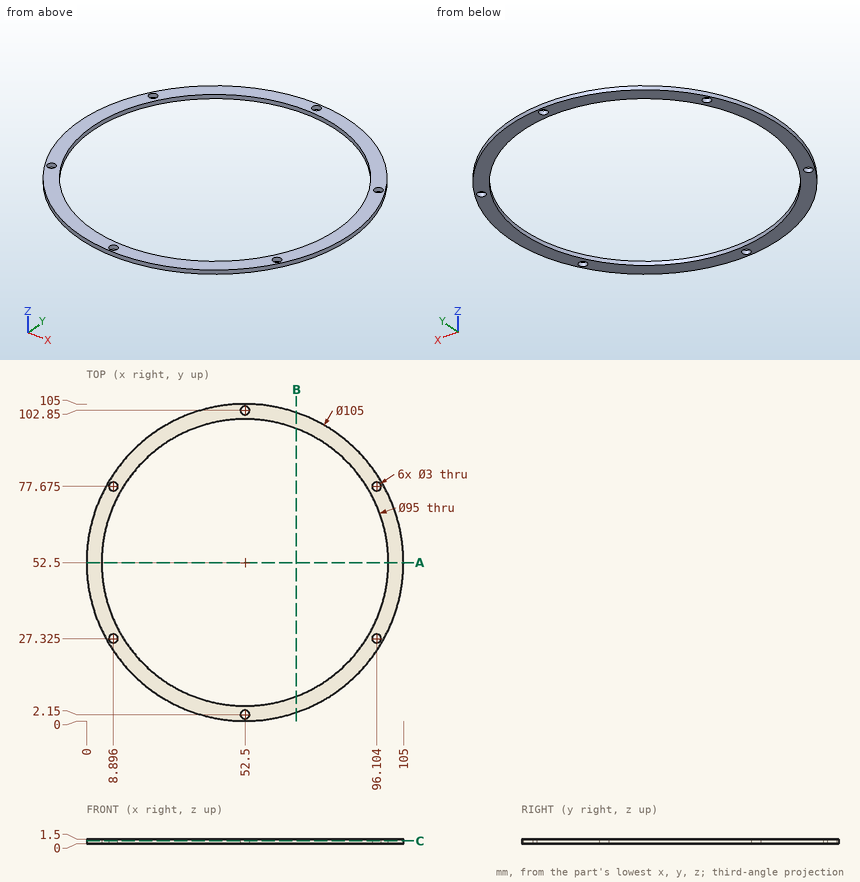
Study the drawing (mm; zero at the part's minimum x, y, z) and answer. Round coordinates to 2 decimals unless told otherwise and drop trailing zeros. Write each loop counter-clockwise with the first axis right and the second up, starting at its lowest first coordinate (ties: lowest second). Pieces come first, ordered by that corner, then holes. Notation, with made-up numbers: (0.25, 41.25) -> (27.25, 41.25) arc R25 ccw to (27.25, 77.25) -> close; hole circle Ø10 at (68, 15.25). An arc over 180 degrees is marked (long way). Write item = value, one per line.
1) Section C-C on z = 0.9 is taken. Give the number of separate pieces and of enclosed holes in the cut face, plus the area to 3 significant figures.
Check values:
separate_pieces = 1
enclosed_holes = 7
area = 1,530 mm²
2) Section A-A on y = 52.5 is taken. Write down the section's boundary in (x, z), plus the area to 3 significant figures.
Check values:
outline = (0, 0) -> (5, 0) -> (5, 1.5) -> (0, 1.5) -> close; (100, 0) -> (105, 0) -> (105, 1.5) -> (100, 1.5) -> close
area = 15.0 mm²
3) Section B-B on x = 69.5 is taken. Write down the section's boundary in (y, z).
Check values:
outline = (2.83, 0) -> (8.15, 0) -> (8.15, 1.5) -> (2.83, 1.5) -> close; (96.85, 0) -> (102.17, 0) -> (102.17, 1.5) -> (96.85, 1.5) -> close
4) Straight lines are drawn through the part: line 1 along Y through (x, z) = (52.5, 1.1); line 2 along X through (y, z) = (51.5, 0.25); line 3 along Y through (x, z) = (51.5, 0.35). For each, find the intervals that lie inside material, in ascending order. Write a range as [from, to].
Check values:
line_1 = [0, 0.65], [3.65, 5], [100, 101.35], [104.35, 105]
line_2 = [0.01, 5.01], [99.99, 104.99]
line_3 = [0.01, 1.03], [3.27, 5.01], [99.99, 101.73], [103.97, 104.99]
5) Given pin 1 (1.8 mm diameter, centred on x = 96.1, y = 27.32, fed in from +Z), flat-ended and moving along its own axis, determine where the tip first touches the part or whether it passes through.
Check values:
pin_1 = through
